from build123d import *

# Parameters (mm, degrees)
SKETCH_1_W          = 110
SKETCH_1_H          = 150
EXTRUDE_1_DEPTH     = 2
CUT_EXTRUDE_1_DEPTH = 187.021504133
FILLET_1_R          = 2
FILLET_2_R          = 2
SKETCH_3_R          = 2
CUT_EXTRUDE_2_DEPTH = 187.021504133
SKETCH_4_R          = 1.5
CUT_EXTRUDE_3_DEPTH = 187.021504133
SKETCH_5_R          = 1.5
CUT_EXTRUDE_4_DEPTH = 187.021504133
SKETCH_6_R          = 7.5
CUT_EXTRUDE_6_DEPTH = 10
CUT_EXTRUDE_7_DEPTH = 10


with BuildPart() as part:
    # 草图1 → 凸台-拉伸1 (new body)
    with BuildSketch(Plane.XY):
        with Locations((55, 75)):
            Rectangle(SKETCH_1_W, SKETCH_1_H)
    extrude(amount=EXTRUDE_1_DEPTH)

    # 草图2 → 切除-拉伸1 (cut, through all)
    with BuildSketch(Plane(origin=(0, 150, 0), x_dir=(1, 0, 0), z_dir=(0, 1, 0))):
        Polygon((0, -2), (0, 0), (2, 0), align=None)
    extrude(amount=-CUT_EXTRUDE_1_DEPTH, mode=Mode.SUBTRACT)

    # 圆角1
    fillet_1_edges = [part.edges().sort_by_distance(p)[0] for p in [
        (1, 150, 1),
    ]]
    fillet(fillet_1_edges, radius=FILLET_1_R)

    # 圆角2
    fillet_2_edges = [part.edges().sort_by_distance(p)[0] for p in [
        (1, 0, 1),
    ]]
    fillet(fillet_2_edges, radius=FILLET_2_R)

    # 草图3 → 切除-拉伸2 (cut, through all)
    with BuildSketch(Plane.XY.offset(2)):
        with Locations((106.2, 47)):
            Circle(SKETCH_3_R)
        with Locations((106.2, 30)):
            Circle(SKETCH_3_R)
        with Locations(Location((106.2, 120, 0), (0, 0, 180))):
            Circle(SKETCH_3_R)
        with Locations(Location((106.2, 103, 0), (0, 0, 180))):
            Circle(SKETCH_3_R)
    extrude(amount=-CUT_EXTRUDE_2_DEPTH, mode=Mode.SUBTRACT)

    # 草图4 → 切除-拉伸3 (cut, through all)
    with BuildSketch(Plane(origin=(0, 0, 0), x_dir=(-1, 0, 0), z_dir=(0, 0, -1))):
        with Locations((-60.760859098, 147)):
            Circle(SKETCH_4_R)
        with Locations((-80.760859098, 147)):
            Circle(SKETCH_4_R)
    extrude(amount=-CUT_EXTRUDE_3_DEPTH, mode=Mode.SUBTRACT)

    # 草图5 → 切除-拉伸4 (cut, through all)
    with BuildSketch(Plane(origin=(0, 0, 0), x_dir=(-1, 0, 0), z_dir=(0, 0, -1))):
        with Locations((-80.76127274, 3)):
            Circle(SKETCH_5_R)
        with Locations((-60.76127274, 3)):
            Circle(SKETCH_5_R)
    extrude(amount=-CUT_EXTRUDE_4_DEPTH, mode=Mode.SUBTRACT)

    # 草图6 → 切除-拉伸6 (cut)
    with BuildSketch(Plane.XY.offset(2)):
        with Locations((15, 135)):
            Circle(SKETCH_6_R)
        with Locations(Location((15, 15, 0), (0, 0, 180))):
            Circle(SKETCH_6_R)
        with Locations((97.828427125, 15)):
            Circle(SKETCH_6_R)
        with Locations(Location((97.828427125, 135, 0), (0, 0, 180))):
            Circle(SKETCH_6_R)
    extrude(amount=-CUT_EXTRUDE_6_DEPTH, mode=Mode.SUBTRACT)

    # 草图7 → 切除-拉伸7 (cut)
    with BuildSketch(Plane.XY.offset(2)):
        with BuildLine():
            Line((56.414213562, 133.123376127), (41.691712888, 139.579112703))
            ThreePointArc((41.691712888, 139.579112703), (35.104684138, 137.007916048), (37.675880793, 130.420887297))
            Line((37.675880793, 130.420887297), (54.406297515, 123.08469044))
            ThreePointArc((54.406297515, 123.08469044), (51.414213562, 127.663803143), (54.406297515, 132.242915846))
            Line((54.406297515, 132.242915846), (56.414213562, 133.123376127))
        make_face()
        with BuildLine():
            Line((58.42212961, 132.242915846), (56.414213562, 133.123376127))
            Line((56.414213562, 133.123376127), (54.406297515, 132.242915846))
            ThreePointArc((54.406297515, 132.242915846), (51.414213562, 127.663803143), (54.406297515, 123.08469044))
            ThreePointArc((54.406297515, 123.08469044), (56.414213562, 122.663803143), (58.42212961, 123.08469044))
            ThreePointArc((58.42212961, 123.08469044), (61.414213562, 127.663803143), (58.42212961, 132.242915846))
        make_face()
        with BuildLine():
            Line((71.136714237, 139.579112703), (56.414213562, 133.123376127))
            Line((56.414213562, 133.123376127), (58.42212961, 132.242915846))
            ThreePointArc((58.42212961, 132.242915846), (61.414213562, 127.663803143), (58.42212961, 123.08469044))
            Line((58.42212961, 123.08469044), (75.152546332, 130.420887297))
            ThreePointArc((75.152546332, 130.420887297), (77.723742987, 137.007916048), (71.136714237, 139.579112703))
        make_face()
        with BuildLine():
            Line((87.859311366, 125.180806839), (56.414213562, 111.787459321))
            Line((56.414213562, 111.787459321), (58.373531952, 110.952930765))
            ThreePointArc((58.373531952, 110.952930765), (61.414213562, 106.352814304), (58.373531952, 101.752697844))
            Line((58.373531952, 101.752697844), (91.777948145, 115.980573918))
            ThreePointArc((91.777948145, 115.980573918), (94.418746216, 122.540008767), (87.859311366, 125.180806839))
        make_face()
        with BuildLine():
            Line((58.373531952, 110.952930765), (56.414213562, 111.787459321))
            Line((56.414213562, 111.787459321), (54.454895173, 110.952930765))
            ThreePointArc((54.454895173, 110.952930765), (51.414213562, 106.352814304), (54.454895173, 101.752697844))
            ThreePointArc((54.454895173, 101.752697844), (56.414213562, 101.352814304), (58.373531952, 101.752697844))
            ThreePointArc((58.373531952, 101.752697844), (61.414213562, 106.352814304), (58.373531952, 110.952930765))
        make_face()
        with BuildLine():
            Line((56.414213562, 111.787459321), (24.969115758, 125.180806839))
            ThreePointArc((24.969115758, 125.180806839), (18.409680909, 122.540008767), (21.05047898, 115.980573918))
            Line((21.05047898, 115.980573918), (54.454895173, 101.752697844))
            ThreePointArc((54.454895173, 101.752697844), (51.414213562, 106.352814304), (54.454895173, 110.952930765))
            Line((54.454895173, 110.952930765), (56.414213562, 111.787459321))
        make_face()
        with BuildLine():
            ThreePointArc((24.969115758, 100.180806839), (18.409680909, 97.540008767), (21.05047898, 90.980573918))
            Line((21.05047898, 90.980573918), (54.454895173, 76.752697844))
            ThreePointArc((54.454895173, 76.752697844), (51.414213562, 81.352814304), (54.454895173, 85.952930765))
            Line((54.454895173, 85.952930765), (56.414213562, 86.787459321))
            Line((56.414213562, 86.787459321), (24.969115758, 100.180806839))
        make_face()
        with BuildLine():
            ThreePointArc((54.454895173, 85.952930765), (51.414213562, 81.352814304), (54.454895173, 76.752697844))
            ThreePointArc((54.454895173, 76.752697844), (56.414213562, 76.352814304), (58.373531952, 76.752697844))
            ThreePointArc((58.373531952, 76.752697844), (61.414213562, 81.352814304), (58.373531952, 85.952930765))
            Line((58.373531952, 85.952930765), (56.414213562, 86.787459321))
            Line((56.414213562, 86.787459321), (54.454895173, 85.952930765))
        make_face()
        with BuildLine():
            ThreePointArc((58.373531952, 85.952930765), (61.414213562, 81.352814304), (58.373531952, 76.752697844))
            Line((58.373531952, 76.752697844), (91.777948145, 90.980573918))
            ThreePointArc((91.777948145, 90.980573918), (94.418746216, 97.540008767), (87.859311366, 100.180806839))
            Line((87.859311366, 100.180806839), (56.414213562, 86.787459321))
            Line((56.414213562, 86.787459321), (58.373531952, 85.952930765))
        make_face()
        with BuildLine():
            ThreePointArc((58.373531952, 60.952930765), (61.414213562, 56.352814304), (58.373531952, 51.752697844))
            Line((58.373531952, 51.752697844), (91.777948145, 65.980573918))
            ThreePointArc((91.777948145, 65.980573918), (94.418746216, 72.540008767), (87.859311366, 75.180806839))
            Line((87.859311366, 75.180806839), (56.414213562, 61.787459321))
            Line((56.414213562, 61.787459321), (58.373531952, 60.952930765))
        make_face()
        with BuildLine():
            ThreePointArc((54.454895173, 60.952930765), (51.414213562, 56.352814304), (54.454895173, 51.752697844))
            ThreePointArc((54.454895173, 51.752697844), (56.414213562, 51.352814304), (58.373531952, 51.752697844))
            ThreePointArc((58.373531952, 51.752697844), (61.414213562, 56.352814304), (58.373531952, 60.952930765))
            Line((58.373531952, 60.952930765), (56.414213562, 61.787459321))
            Line((56.414213562, 61.787459321), (54.454895173, 60.952930765))
        make_face()
        with BuildLine():
            ThreePointArc((24.969115758, 75.180806839), (18.409680909, 72.540008767), (21.05047898, 65.980573918))
            Line((21.05047898, 65.980573918), (54.454895173, 51.752697844))
            ThreePointArc((54.454895173, 51.752697844), (51.414213562, 56.352814304), (54.454895173, 60.952930765))
            Line((54.454895173, 60.952930765), (56.414213562, 61.787459321))
            Line((56.414213562, 61.787459321), (24.969115758, 75.180806839))
        make_face()
        with BuildLine():
            ThreePointArc((24.969115758, 50.180806839), (18.409680909, 47.540008767), (21.05047898, 40.980573918))
            Line((21.05047898, 40.980573918), (54.454895173, 26.752697844))
            ThreePointArc((54.454895173, 26.752697844), (51.414213562, 31.352814304), (54.454895173, 35.952930765))
            Line((54.454895173, 35.952930765), (56.414213562, 36.787459321))
            Line((56.414213562, 36.787459321), (24.969115758, 50.180806839))
        make_face()
        with BuildLine():
            ThreePointArc((54.454895173, 35.952930765), (51.414213562, 31.352814304), (54.454895173, 26.752697844))
            ThreePointArc((54.454895173, 26.752697844), (56.414213562, 26.352814304), (58.373531952, 26.752697844))
            ThreePointArc((58.373531952, 26.752697844), (61.414213562, 31.352814304), (58.373531952, 35.952930765))
            Line((58.373531952, 35.952930765), (56.414213562, 36.787459321))
            Line((56.414213562, 36.787459321), (54.454895173, 35.952930765))
        make_face()
        with BuildLine():
            ThreePointArc((58.373531952, 35.952930765), (61.414213562, 31.352814304), (58.373531952, 26.752697844))
            Line((58.373531952, 26.752697844), (91.777948145, 40.980573918))
            ThreePointArc((91.777948145, 40.980573918), (94.418746216, 47.540008767), (87.859311366, 50.180806839))
            Line((87.859311366, 50.180806839), (56.414213562, 36.787459321))
            Line((56.414213562, 36.787459321), (58.373531952, 35.952930765))
        make_face()
        with BuildLine():
            ThreePointArc((58.42212961, 17.242915846), (61.414213562, 12.663803143), (58.42212961, 8.08469044))
            Line((58.42212961, 8.08469044), (75.152546332, 15.420887297))
            ThreePointArc((75.152546332, 15.420887297), (77.723742987, 22.007916048), (71.136714237, 24.579112703))
            Line((71.136714237, 24.579112703), (56.414213562, 18.123376127))
            Line((56.414213562, 18.123376127), (58.42212961, 17.242915846))
        make_face()
        with BuildLine():
            ThreePointArc((54.406297515, 17.242915846), (51.414213562, 12.663803143), (54.406297515, 8.08469044))
            ThreePointArc((54.406297515, 8.08469044), (56.414213562, 7.663803143), (58.42212961, 8.08469044))
            ThreePointArc((58.42212961, 8.08469044), (61.414213562, 12.663803143), (58.42212961, 17.242915846))
            Line((58.42212961, 17.242915846), (56.414213562, 18.123376127))
            Line((56.414213562, 18.123376127), (54.406297515, 17.242915846))
        make_face()
        with BuildLine():
            ThreePointArc((41.691712888, 24.579112703), (35.104684138, 22.007916048), (37.675880793, 15.420887297))
            Line((37.675880793, 15.420887297), (54.406297515, 8.08469044))
            ThreePointArc((54.406297515, 8.08469044), (51.414213562, 12.663803143), (54.406297515, 17.242915846))
            Line((54.406297515, 17.242915846), (56.414213562, 18.123376127))
            Line((56.414213562, 18.123376127), (41.691712888, 24.579112703))
        make_face()
    extrude(amount=-CUT_EXTRUDE_7_DEPTH, mode=Mode.SUBTRACT)


solid = part.part
Verification items for the finished model (mm, model axes). Give positions to 0.01 mm unless a question says otherwise; leave off trailing zeros. Write each loop counter-clockwise with the first axis right and the second up, starting at its lowest first coordinate (ties: lowest second). Pieces come first, ordered by that corner, then holes.
(1) Material ranges on line 1 (Y direction, x = 15, z = 0.65); line 2 (Y direction, x = 106.2, z = 1.35); line 3 (Y direction, x = 25, z = 1.05), recorded low to high.
(2) Cross-section at B-B (y = 120). Enter the section's corners in (x, z).
(3) Cross-section at A-A (x = 15). Enter the section's corners in (y, z), plus the area to 3 significant figures.
(4) Cross-section at C-C (x = 67.5). Enter the section's corners in (y, z).
(5) Gauge pin test, flat end, axial feed: pin 1 (17 mm diameter, centred on x = 15, y = 135, fed in from +Z). Record the tip position at first contact, or that the pin passes through.
(6) Cross-section at D-D (y = 69). Enter the section's corners in (x, z), plus the area to 3 significant figures.
Worked out:
1. line 1: y = 0 to 7.5, 22.5 to 127.5, 142.5 to 150
1. line 2: y = 0 to 28, 32 to 45, 49 to 101, 105 to 118, 122 to 150
1. line 3: y = 0 to 39.3, 50.17 to 64.3, 75.17 to 89.3, 100.17 to 114.3, 125.17 to 150
2. outline: (0, 2) - (2, 0) - (18.04, 0) - (18.04, 2) - close; (37.13, 0) - (75.7, 0) - (75.7, 2) - (37.13, 2) - close; (94.78, 0) - (104.2, 0) - (104.2, 2) - (94.78, 2) - close; (108.2, 0) - (110, 0) - (110, 2) - (108.2, 2) - close
3. outline: (0, 0) - (7.5, 0) - (7.5, 2) - (0, 2) - close; (22.5, 0) - (127.5, 0) - (127.5, 2) - (22.5, 2) - close; (142.5, 0) - (150, 0) - (150, 2) - (142.5, 2) - close
3. area: 240 mm2
4. outline: (0, 0) - (12.07, 0) - (12.07, 2) - (0, 2) - close; (22.98, 0) - (30.64, 0) - (30.64, 2) - (22.98, 2) - close; (41.51, 0) - (55.64, 0) - (55.64, 2) - (41.51, 2) - close; (66.51, 0) - (80.64, 0) - (80.64, 2) - (66.51, 2) - close; (91.51, 0) - (105.64, 0) - (105.64, 2) - (91.51, 2) - close; (116.51, 0) - (127.07, 0) - (127.07, 2) - (116.51, 2) - close; (137.98, 0) - (150, 0) - (150, 2) - (137.98, 2) - close
5. pin 1: stops at z = 2
6. outline: (0, 2) - (2, 0) - (18.27, 0) - (18.27, 2) - close; (39.48, 0) - (73.35, 0) - (73.35, 2) - (39.48, 2) - close; (94.56, 0) - (110, 0) - (110, 2) - (94.56, 2) - close
6. area: 133 mm2
